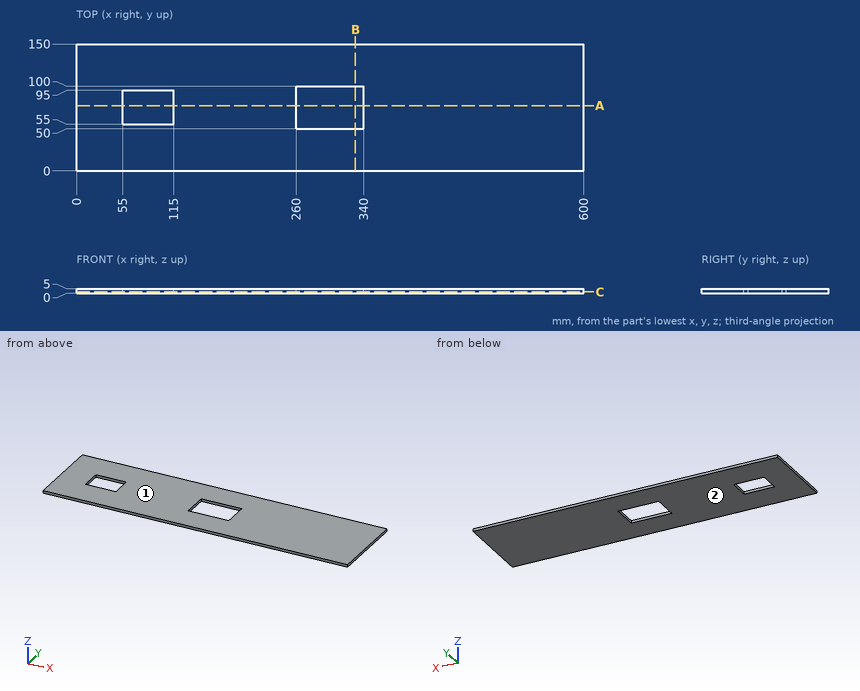
Design review of the part shown in the three views and the two pictorial views. Dimensions are in mm from the part's minimum x, y and z. Round coordinates to 2 decimals unless told otherwise and drop trailing zeros. Write each loop counter-clockwise with the first axis right and the second up, starting at its lowest first coordinate (ties: lowest second). Pieces come first, ordered by that corner, then holes. Notation, with made-up numbers: M 41.5,-1 L 51.5,-1 A15 cw 51.5,26 Z; hole C -16.5,36 d1. An arc over 180 degrees is marked long. One line per item, written item: value. Start each with the question number.
1. To check wall thickness, follow probe 1 along X at (y, z) = (94, 2.7); probe 2 along X at (y, z) = (98, 4.1); probe 3 along Y at (x, z) = (314.5, 1.75). State the ranges of each line that lie inside material, in increasing order. Write a range as from..to.
2. Take a section at C-C on z = 1.4. State the section outline as (x, y) points.
3. Take a section at A-A on y = 77. State the section outline as (x, z) points, then the cut area to 3 significant figures.
4. Take a section at B-B on x = 330. State the section outline as (y, z) points, then the cut area to 3 significant figures.
5. Draft analysis for pull direction Z (two halves, no side actions). For the marked faces 1 and 2, state which applies: pulls with the +Z half, pulls with the -Z half, needs draft (parallel to the pull), parting line crosses it, or undercut.
Computed:
1. probe 1: x = 0..55, 115..260, 340..600
1. probe 2: x = 0..260, 340..600
1. probe 3: y = 0..50, 100..150
2. outline: M 0,0 L 600,0 L 600,150 L 0,150 Z; hole M 55,55 L 115,55 L 115,95 L 55,95 Z; hole M 260,50 L 340,50 L 340,100 L 260,100 Z
3. outline: M 0,0 L 55,0 L 55,5 L 0,5 Z; M 115,0 L 260,0 L 260,5 L 115,5 Z; M 340,0 L 600,0 L 600,5 L 340,5 Z
3. area: 2,300 mm²
4. outline: M 0,0 L 50,0 L 50,5 L 0,5 Z; M 100,0 L 150,0 L 150,5 L 100,5 Z
4. area: 500 mm²
5. face 1: pulls with the +Z half
5. face 2: pulls with the -Z half
